```python
from build123d import *

# Parameters (mm, degrees)
SKETCH1_W               = 100
SKETCH1_H               = 70
BOSS_EXTRUDE1_DEPTH     = 20
CUT_EXTRUDE1_DEPTH      = 73.972597597
CUT_EXTRUDE1_DEPTH_BACK = 73.972597597
SKETCH2_R               = 9.1
CUT_EXTRUDE2_DEPTH      = 108.819293264
CUT_EXTRUDE2_DEPTH_BACK = 108.819293264
SKETCH3_R               = 9.1
SKETCH4_R               = 2.6
CUT_EXTRUDE4_DEPTH      = 20
SKETCH5_W               = 100
SKETCH5_H               = 20
BOSS_EXTRUDE2_DEPTH     = 20


with BuildPart() as part:
    # Sketch1 → Boss-Extrude1 (new, symmetric)
    with BuildSketch(Plane.XY):
        Rectangle(SKETCH1_W, SKETCH1_H)
    extrude(amount=BOSS_EXTRUDE1_DEPTH, both=True)

    # Sketch2 → Cut-Extrude1 (cut, two sides: drawn at the far end of the back side and taken through both)
    with BuildSketch(Plane.XY.offset(20).offset(-CUT_EXTRUDE1_DEPTH_BACK)):
        with Locations((25, 17.5)):
            Circle(SKETCH2_R)
        with Locations((-25, 17.5)):
            Circle(SKETCH2_R)
    extrude(amount=CUT_EXTRUDE1_DEPTH + CUT_EXTRUDE1_DEPTH_BACK, mode=Mode.SUBTRACT)

    # Sketch3 → Cut-Extrude2 (cut, two sides: drawn at the far end of the back side and taken through both)
    with BuildSketch(Plane.ZY.offset(50).offset(-CUT_EXTRUDE2_DEPTH_BACK)):
        with Locations((0, -17.5)):
            Circle(SKETCH3_R)
    extrude(amount=CUT_EXTRUDE2_DEPTH + CUT_EXTRUDE2_DEPTH_BACK, mode=Mode.SUBTRACT)

    # Sketch4 → Cut-Extrude4 (cut)
    with BuildSketch(Plane(origin=(0, 35, 0), x_dir=(1, 0, 0), z_dir=(0, 1, 0))):
        with Locations(Location((-25, 0, 0), (0, 0, 270))):
            Circle(SKETCH4_R)
        with Locations(Location((25, 0, 0), (0, 0, 270))):
            Circle(SKETCH4_R)
    extrude(amount=-CUT_EXTRUDE4_DEPTH, mode=Mode.SUBTRACT)

    # Sketch5 → Boss-Extrude2 (add)
    with BuildSketch(Plane.XZ.offset(35)):
        Rectangle(SKETCH5_W, SKETCH5_H)
    extrude(amount=BOSS_EXTRUDE2_DEPTH)


solid = part.part
```
Verification items for the finished model (mm, model axes). A direction names the side the tool comes from. Round coordinates to 2 decimals unless told otherwise and drop trailing zeros. Order: outer loops, then holes, each group sorted by start corner. A loop starts at its lowest first (then second) coordinate and runs counter-clockwise, first axis right, second up. Notation, with made-up numbers: (48, 81.25) - (93, 81.25) arc R16 cw to (93, 99.25) - close; hole circle Ø9 at (-36, 76). An arc over 180 degrees is marked (long way). Use CSV: the item, a comma, the result in double quotes. Start each with the question number.
1) Section check A-A, the plane x = 25. Record the cut outline in (y, z).
2) Thickness scan on L1, parallel to X at y = 17.5, z = -10; L2, parallel to X at y = 28.5, z = 0; L3, parallel to Y at x = -30, z = 0. Record the ranges inside material, lowest first.
3) Mould release check, pull along Y, two halves, no side actions. Record for faces 6 (the flat face through (-1, -45, -10)), 7 (the cylindrical face through (-20.801, 9.427, -0.28)), 8 (the flat face through (-1, -35, 15)): +Y half, -Y half, draft (parallel to the pull), parting line (faces both ways), or undercut.
4) Access from +Z, -Z, +X, -X, +Y, -Y to the whole of each face (thin tool, end or side, straight path). Record for faces 1 (the cylindrical face through (29.199, 9.427, -0.28)), 2 (the flat face through (-1, -35, -15)), 3 (the cylindrical face through (-22.422, 30.672, -0.338)), 4 (the flat face through (-1, -45, 10)), 5 (the flat face through (-50, -1, 0)).
5) Section check D-D, the plane y = 17.5. Record the cut outline in (x, z).
6) Section check B-B, the plane z = 0. Record the cut outline in (x, y).
7) Go/stop test with flat-tipped pins: P1, Ø10, axis at y = -23.5, z = 3.5, coming from the -X side; P2, Ø16, axis at x = 6, y = -43.5, coming from the +Z side; P3, Ø3, axis at x = -18.5, z = -14, coming from the -Y side; P4, Ø5, axis at x = -13.5, y = -45, coming from the -Z side. Record where each tip stops, or that it passes through.
8) Section check C-C, the plane y = -17.5. Record the cut outline in (x, z), plus the area to 3 significant figures.
Answers:
1,outline,"(-55, -10) - (-35, -10) - (-35, -20) - (8.4, -20) - (8.4, 20) - (-35, 20) - (-35, 10) - (-55, 10) - close; (26.6, -20) - (35, -20) - (35, -2.6) - (26.6, -2.6) - close; (26.6, 2.6) - (35, 2.6) - (35, 20) - (26.6, 20) - close; hole circle Ø18.2 at (-17.5, 0)"
2,L1,"x = -50 to -34.1, -15.9 to 15.9, 34.1 to 50"
2,L2,"x = -50 to -27.6, -22.4 to 22.4, 27.6 to 50"
2,L3,"y = -55 to -26.6, -8.4 to 9.9, 25.1 to 35"
3,face 6,"draft"
3,face 7,"undercut"
3,face 8,"-Y half"
4,face 1,"+Z, -Z"
4,face 2,"-Z, +X, -X, -Y"
4,face 3,"+Y"
4,face 4,"+Z, +X, -X, -Y"
4,face 5,"+Z, -Z, -X, +Y, -Y"
5,outline,"(-50, -20) - (-34.1, -20) - (-34.1, 20) - (-50, 20) - close; (-15.9, -20) - (15.9, -20) - (15.9, 20) - (-15.9, 20) - close; (34.1, -20) - (50, -20) - (50, 20) - (34.1, 20) - close"
6,outline,"(-50, -55) - (50, -55) - (50, -26.6) - (-50, -26.6) - close; (-50, -8.4) - (50, -8.4) - (50, 35) - (27.6, 35) - (27.6, 26.22) arc R9.1 cw (long way) to (22.4, 26.22) - (22.4, 35) - (-22.4, 35) - (-22.4, 26.22) arc R9.1 cw (long way) to (-27.6, 26.22) - (-27.6, 35) - (-50, 35) - close"
7,P1,"stops at x = -50"
7,P2,"stops at z = 10"
7,P3,"stops at y = -35"
7,P4,"stops at z = -10"
8,outline,"(-50, -20) - (50, -20) - (50, -9.1) - (-50, -9.1) - close; (-50, 9.1) - (50, 9.1) - (50, 20) - (-50, 20) - close"
8,area,"2,180 mm²"
